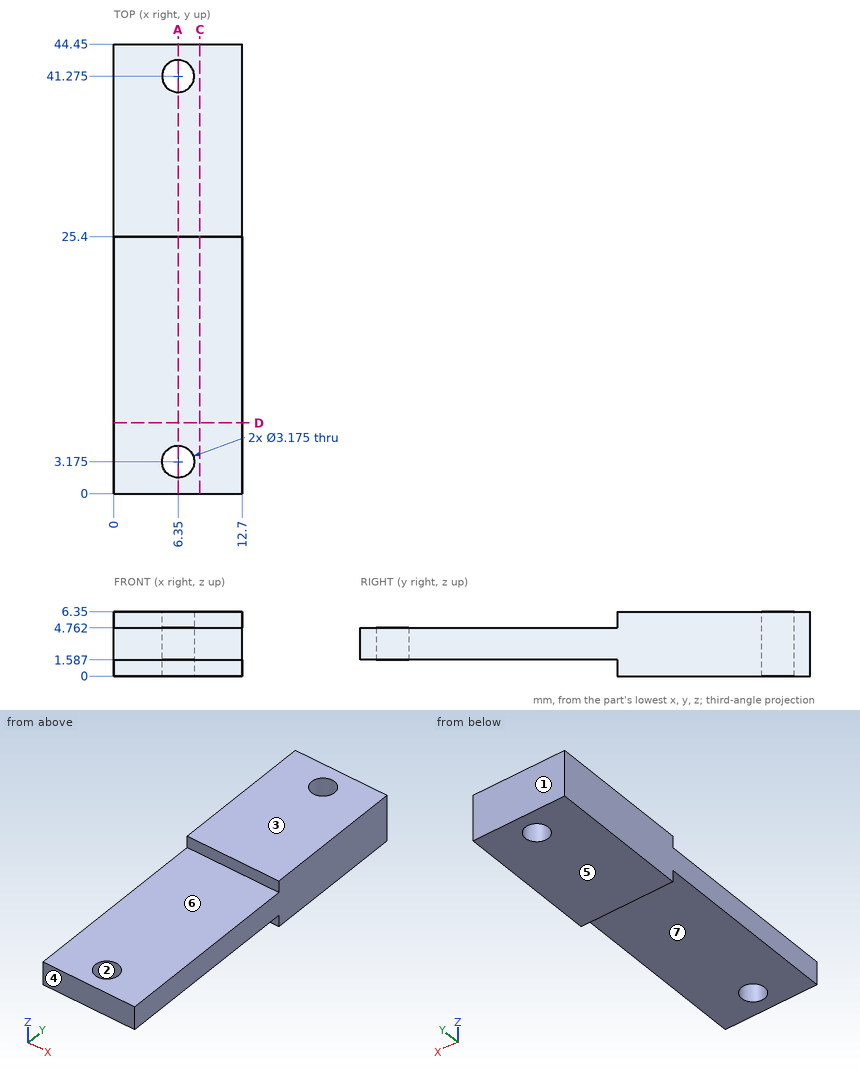
Geometry check sheet. Reference: drawing and pictorial views, mm from the part's lowest x, y, z. A direction names the side the tool comes from. Round coordinates to 2 decimals unless told otherwise and drop trailing zeros. Loops run counter-clockwise (first coordinate to the right, second up) from the corner with the lowest first, then second, coordinate; pieces in that order, holes last. Notation, with made-up numbers: (16.25, 11) - (75.25, 11) arc R30 cw to (75.25, 34) - close; hole circle Ø6 at (-24.5, 46). An arc over 180 degrees is marked (long way). Write item = value, one per line. Start each with the question number.
Q1. Depth check by flat-ended pin: P1, Ø5, axis at x = 5, y = 22.5, coming from the -Z side; P2, Ø1.9, axis at x = 6.35, y = 3.175, coming from the -Z side. Enter the tip coordinate at first touch or a pass-through.
Q2. Section check A-A (x = 6.35). Record the boundary of the cut face in (y, z).
Q3. Section check D-D (y = 7). Record the boundary of the cut face in (x, z).
Q4. Section check C-C (x = 8.5). Record the boundary of the cut face in (y, z), plus the area to 3 significant figures.
Q5. Thickness scan on L1, parallel to Y at x = 6.35, z = 2.5; L2, parallel to Y at x = 7.5, z = 2.5; L3, parallel to Z at x = 6, y = 22. Record the ranges inside material, lowest first.
Q6. Access from +Z, -Z, +X, -X, +Y, -Y to the whole of each face (thin tool, end or side, straight path). Record for the marked faces 5, 6 and 7.
Q7. Release check for a two-part mould opening along Y. For the marked faces 1, 2, 3 and 4 record: pulls with the +Y half, pulls with the -Y half, needs draft (parallel to the pull), parting line crosses it, or undercut.
Derived:
q1.P1 = 1.59
q1.P2 = through
q2.outline = (0, 1.59) - (1.59, 1.59) - (1.59, 4.76) - (0, 4.76) - close; (4.76, 1.59) - (25.4, 1.59) - (25.4, 0) - (39.69, 0) - (39.69, 6.35) - (25.4, 6.35) - (25.4, 4.76) - (4.76, 4.76) - close; (42.86, 0) - (44.45, 0) - (44.45, 6.35) - (42.86, 6.35) - close
q3.outline = (0, 1.59) - (12.7, 1.59) - (12.7, 4.76) - (0, 4.76) - close
q4.outline = (0, 1.59) - (25.4, 1.59) - (25.4, 0) - (44.45, 0) - (44.45, 6.35) - (25.4, 6.35) - (25.4, 4.76) - (0, 4.76) - close
q4.area = 202 mm^2
q5.L1 = 0 to 1.59, 4.76 to 39.69, 42.86 to 44.45
q5.L2 = 0 to 2.08, 4.27 to 40.18, 42.37 to 44.45
q5.L3 = 1.59 to 4.76
q6.face_5 = -Z, +X, -X, +Y, -Y
q6.face_6 = +Z, +X, -X, -Y
q6.face_7 = -Z, +X, -X, -Y
q7.face_1 = pulls with the +Y half
q7.face_2 = undercut
q7.face_3 = needs draft
q7.face_4 = pulls with the -Y half
